Can you work these out from the drawing? Everything is in mm from the part's minimum corner. Round coordinates to 2 decimals unless told otherwise and drop trailing zeros. Loops run counter-clockwise (first coordinate to the right, second up) from the corner with the lowest first, then second, coordinate; pieces in that order, holes last. Notation, with made-up numbers: (66, 22) -> (90, 22) arc R34 ccw to (90, 59) -> close; hole circle Ø6 at (-0.5, 59.5). An arc over 180 degrees is marked (long way). One line per item, written item: value.
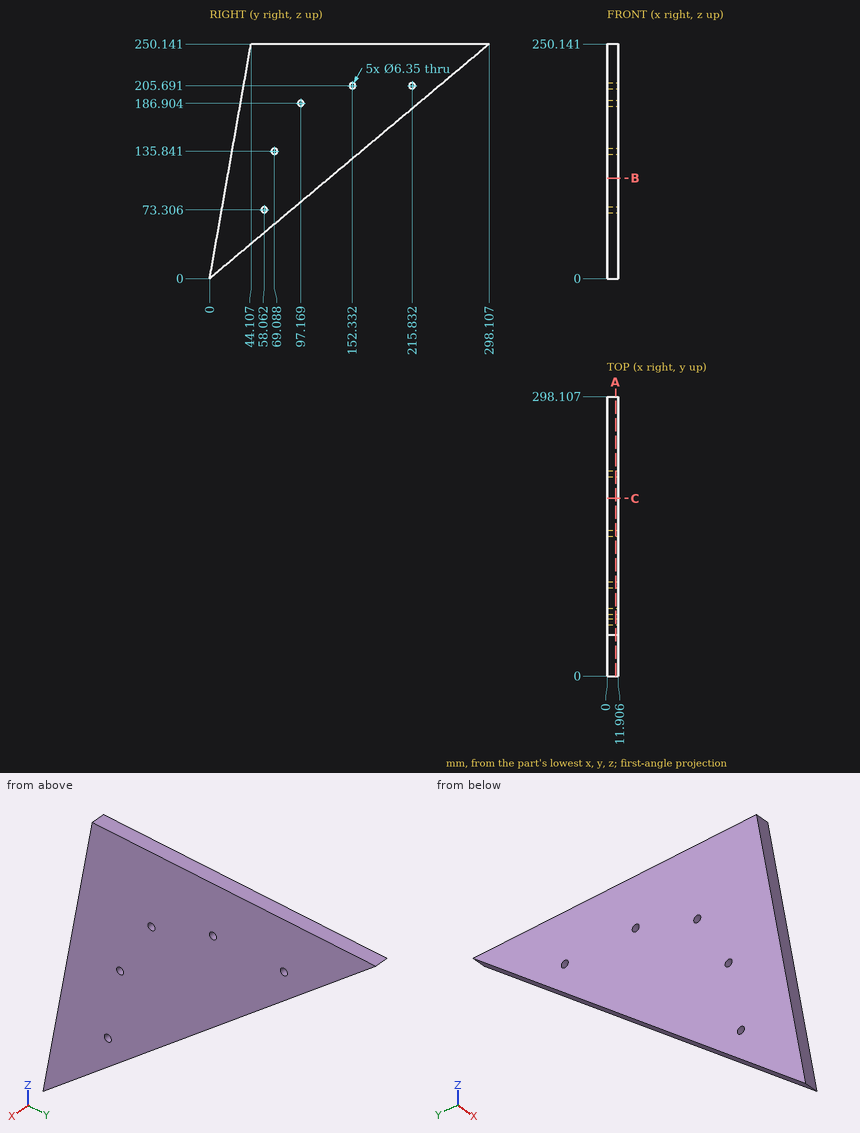
Item 1: I need wall thicknesses on line 1 (Z direction, x = 8.25, y = 112); line 2 (Z direction, x = 11, y = 214) (1 decimal); line 3 (Y direction, x = 5, z = 211) (1 decimal). Which ranges of each line are inside material? Lowest first, please. Write a range as from..to.
Output:
line 1: z = 93.98..250.14
line 2: z = 179.6..203.1, 208.3..250.1
line 3: y = 37.2..251.5
Item 2: If we section it at A-A on x = 9: Count the separate pieces of the cut face and the enclosed holes in it, plus the area to 3 significant figures.
Output:
separate pieces: 1
enclosed holes: 5
area: 31,600 mm²
Item 3: If we section it at C-C on y = 189.5: List the corners of the cut face in (x, z) for me.
Output:
outline: (0, 159.01) -> (11.91, 159.01) -> (11.91, 250.14) -> (0, 250.14) -> close
Item 4: Will these pins go through, and if not, where does the flat tip stop? pin 1 Ø5 at (y, z) = (69.09, 135.84) entering from +X; pin 2 Ø2 at (x, z) = (6.5, 34) entering from -Y; pin 3 Ø5 at (x, z) = (6.5, 172) entering from +Y; pin 4 Ø6 at (x, y) = (5, 93.5) entering from -Z.
Output:
pin 1: passes through
pin 2: stops at y = 5.82
pin 3: stops at y = 207.96
pin 4: stops at z = 75.94
Item 5: If we section it at B-B on z = 107: List the corners of the cut face in (x, y) for me, plus the area to 3 significant figures.
Output:
outline: (0, 18.87) -> (11.91, 18.87) -> (11.91, 127.52) -> (0, 127.52) -> close
area: 1,290 mm²
